Work out the finished part from the listing and answer in its coordinate system (mm). A direction names the side the tool comes from. Round coordinates to 2 decimals unless told otherwise and drop trailing zeros. Loops run counter-clockwise (first coordinate to the right, second up) from the corner with the lowest first, then second, coordinate; pieces in that order, holes last. Notation, with made-up numbers: M 4.25,62.25 L 49.25,62.25 A21 cw 49.25,96.25 Z; hole C 76.25,40 d3. An arc over 180 degrees is marked long. One line per item, written item: value.
```python
from build123d import *

# Parameters (mm, degrees)
FILLET1_R   = 0.2
HEX_START   = -1.5
HEX_2_DEPTH = 1.5


with BuildPart() as part:
    # BodySke → BaseBody (revolve)
    with BuildSketch(Plane.XY, mode=Mode.PRIVATE) as basebody_sk:
        Polygon((0, 0), (0, 3.9), (0.58, 3.9), (2.48, 2), (29.61, 2), (30, 1.61), (30, 0), align=None)
    revolve(basebody_sk.sketch.rotate(Axis((0, 0, 0), (1, 0, 0)), 90), axis=Axis((0, 0, 0), (1, 0, 0)))

    # Fillet1
    fillet1_edges = [part.edges().sort_by_distance(p)[0] for p in [
        (2.48, 0, -2),
    ]]
    fillet(fillet1_edges, radius=FILLET1_R)

    # Hex 2: read off the stored shape, not the designer's step
    # Hex 2 outline → Hex 2 (cut)
    with BuildSketch(Plane.ZY.offset(HEX_START)):
        Polygon((-1.25, -0.721687836), (0, -1.443375673), (1.25, -0.721687836), (1.25, 0.721687836), (0, 1.443375673), (-1.25, 0.721687836), align=None)
    extrude(amount=HEX_2_DEPTH, mode=Mode.SUBTRACT)

    # Hex 2 2 outline → Hex 2 2 (revolve, cut)
    with BuildSketch(Plane.YX):
        Polygon((1.25, 1.5), (0, 2.221687836), (0, 1.5), align=None)
    revolve(axis=Axis((0, 0, 0), (1, 0, 0)), mode=Mode.SUBTRACT)


solid = part.part
```
1) For faces 5 (the face through (16, 2, 0)), 6 (the face through (30, 0, 0)), 7 (the face through (1, 0, -1.25)), determine the directions among +Z, -Z, +X, -X, +Y, -Y from which every point of the face is accessible in a straight line to the end or side of a thin tool.
Check values:
face 5: +X
face 6: +Z, -Z, +X, +Y, -Y
face 7: -X
2) The mould has two halves that part along Y. Classify faces 1 (the face through (0, 0, -2)), 2 (the face through (0.76, -1.08, -0.63)), 3 (the face through (2.106, -0.199, 0.009)), 4 (the face through (0.29, -2.64, -2.87)): +Y half, -Y half, draft (parallel to the pull), parting line (faces both ways), or undercut.
Check values:
face 1: draft
face 2: undercut
face 3: undercut
face 4: parting line
3) Find the intervals of material crossed by probe 1 along X at (y, z) = (3.5, -1.25); probe 2 along Z at (x, y) = (2.5, 0.5); probe 3 along X at (y, z) = (3.25, -1.25), in increasing order. Write a range as from..to.
Check values:
probe 1: 0..0.76
probe 2: -1.95..1.95
probe 3: 0..1
4) Each of these flat-tipped pins is pushed along its axis until it touches: pin 1 (0.7 mm diameter, centred on y = 0.5, z = 1, fed in from -X); pin 2 (2 mm diameter, centred on x = 25.5, z = -1.5, fed in from +Y); pin 3 (2 mm diameter, centred on x = 15.5, y = -2, fed in from -Z); pin 4 (4 mm diameter, centred on x = 21, z = -2, fed in from -Y). Where does it stop, or does it pass through?
Check values:
pin 1: x = 0
pin 2: y = 1.94
pin 3: z = -1.73
pin 4: y = -2
5) Find section A-A (x = 6.75). Give the vertices of the cut face in (y, z), then the cut area to 3 significant figures.
Check values:
outline: C 0,0 d4
area: 12.6 mm2
